Design review of the part built by this model. Coordinates are the model's own, in mm. Give positions to 0.01 mm unless a question says otherwise; leave off trailing zeros. Write each loop counter-clockwise with the first axis right and the second up, starting at its lowest first coordinate (ties: lowest second). Pieces come first, ordered by that corner, then holes. Notation, with made-up numbers: (-25, 31) -> (-19, 31) arc R27 ccw to (-19, 59) -> close; hole circle Ø11 at (33.25, 10). An arc over 180 degrees is marked (long way). Put each result on its own line as item: value. Start each with the question number.
from build123d import *

# Parameters (mm, degrees)
F1_DEPTH = 4.7625
F3_D     = 12.7
F4_R     = 31.75


# Not quite as in the source:
# - a length typed as a fraction of an inch, garbled in the dataset ("3 / 203.2 mm" for 3/8 in), is restored


with BuildPart() as f1:
    # F0 (on Front) → F1 (new body, symmetric)
    with BuildSketch(Plane.XZ):
        with BuildLine():
            Line((31.75, -36.5125), (31.75, 36.5125))
            Line((31.75, 36.5125), (-31.75, 36.5125))
            Line((-31.75, 36.5125), (-31.75, -36.5125))
            Line((-31.75, -36.5125), (13.9433553622, -74.3740279097))
            ThreePointArc((13.9433553622, -74.3740279097), (19.5317526148, -53.0254697777), (36.0181289039, -38.3560964092))
            Line((36.0181289039, -38.3560964092), (31.75, -36.5125))
        make_face()
        with BuildLine():
            Line((62.0881194933, -49.616895256), (36.0181289039, -38.3560964092))
            ThreePointArc((36.0181289039, -38.3560964092), (19.5317526148, -53.0254697777), (13.9433553622, -74.3740279097))
            Line((13.9433553622, -74.3740279097), (35.8101662485, -92.4928739454))
            ThreePointArc((35.8101662485, -92.4928739454), (73.672422944, -86.207359662), (62.0881194933, -49.616895256))
        make_face()
        with BuildLine():
            ThreePointArc((48.5832224491, -34.9895780081), (42.1559369458, -36.1326186582), (36.0181289039, -38.3560964092))
            Line((36.0181289039, -38.3560964092), (62.0881194933, -49.616895256))
            ThreePointArc((62.0881194933, -49.616895256), (73.672422944, -86.207359662), (35.8101662485, -92.4928739454))
            Line((35.8101662485, -92.4928739454), (13.9433553622, -74.3740279097))
            ThreePointArc((13.9433553622, -74.3740279097), (16.6920555351, -87.2110882282), (23.6346841746, -98.3531426993))
            ThreePointArc((23.6346841746, -98.3531426993), (65.6226967812, -108.5221298326), (90.1161548124, -72.9346037083))
            ThreePointArc((90.1161548124, -72.9346037083), (77.7145523982, -44.8062841439), (48.5832224491, -34.9895780081))
        make_face()
        with BuildLine():
            Line((13.9433553622, -74.3740279097), (-31.75, -36.5125))
            Line((-31.75, -36.5125), (23.6346841746, -98.3531426993))
            ThreePointArc((23.6346841746, -98.3531426993), (16.6920555351, -87.2110882282), (13.9433553622, -74.3740279097))
        make_face()
        with BuildLine():
            Line((48.5832224491, -34.9895780081), (31.75, -36.5125))
            Line((31.75, -36.5125), (36.0181289039, -38.3560964092))
            ThreePointArc((36.0181289039, -38.3560964092), (42.1559369458, -36.1326186582), (48.5832224491, -34.9895780081))
        make_face()
    extrude(amount=F1_DEPTH, both=True)

    # F3 (through all)
    with Locations(Plane.XZ.offset(4.7625)):
        with Locations((52.0161548124, -72.9346037083)):
            Hole(F3_D / 2)

    # F4
    f4_edges = [f1.edges().sort_by_distance(p)[0] for p in [
        (-31.75, 0, -36.5125),
        (31.75, 0, -36.5125),
    ]]
    fillet(f4_edges, radius=F4_R)


solid = f1.part
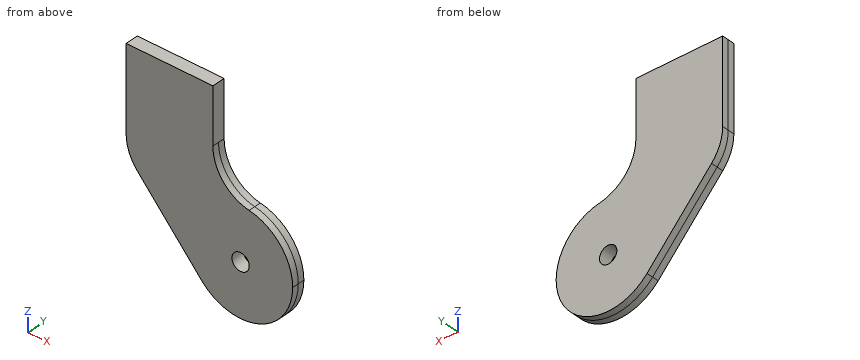
Q1. Take a section at B-B on x = 2. Give the boundary of the cut face in (y, z).
Q2. Take a section at A-A on z = 16. Give the boundary of the cut face in (x, y), then the cut area to 3 significant figures.
Q3. To check wall thickness, follow probe 1 along Z at (x, y) = (50.5, -4); probe 2 along X at (y, z) = (-2.5, 8); probe 3 along X at (y, z) = (1.5, -71). State the ranges of each line that lie inside material, in increasing order. Write a range as from..to.
Q4. For pin 1 (16.5 mm diameter, centred on x = 52.02, z = -72.93, fed in from +Y); pin 2 (3 mm diameter, centred on y = 3.5, z = -0.5, fed in from +X); pin 3 (1 mm diameter, centred on y = 0.5, z = -68.5, fed in from -X); pin 4 (2 mm diameter, centred on x = 75.5, y = 0.5, fed in from +Z), all flat-tipped, find the tip position at first contact; note any pin that passes through.
Result:
1. outline: (-4.76, -74.2) -> (4.76, -74.2) -> (4.76, 36.51) -> (-4.76, 36.51) -> close
2. outline: (-31.75, -4.76) -> (31.75, -4.76) -> (31.75, 4.76) -> (-31.75, 4.76) -> close
2. area: 605 mm^2
3. probe 1: z = -111..-79.1, -66.77..-33
3. probe 2: x = -31.75..31.75
3. probe 3: x = -0.86..45.97, 58.06..90.07
4. pin 1: stops at y = 4.76
4. pin 2: stops at x = 31.75
4. pin 3: stops at x = -3.55
4. pin 4: stops at z = -42.18
